from build123d import *

# Parameters (mm, degrees)
F1_DEPTH = 5
F3_DEPTH = 3
F4_W     = 12
F4_H     = 8
F5_DEPTH = 3.5
F6_W     = 12
F6_H     = 8
F7_DEPTH = 2
F8_W     = 11.5
F8_H     = 1
F9_DEPTH = 2


with BuildPart() as f1:
    # F0 (on Top) → F1 (new body)
    with BuildSketch(Plane.XY):
        Polygon((-20, -5), (-20, -15), (20, -15), (20, -5), (50, -5), (50, 5), (20, 5), (20, 15), (-20, 15), (-20, 5), (-50, 5), (-50, -5), align=None)
    extrude(amount=F1_DEPTH)

    # F2 (on face) → F3 (cut)
    with BuildSketch(Plane.XY.offset(5)):
        Polygon((16.5, 11), (-16.5, 11), (-16.5, 4), (-14.5, 4), (-14.5, -4), (-16.5, -4), (-16.5, -11), (16.5, -11), (16.5, -4), (14.5, -4), (14.5, 4), (16.5, 4), align=None)
    extrude(amount=-F3_DEPTH, mode=Mode.SUBTRACT)

    # F4 (on face) → F5 (cut)
    with BuildSketch(Plane.XY.offset(5)):
        with Locations((-20.5, 0)):
            Rectangle(F4_W, F4_H)
        with Locations((20.5, 0)):
            Rectangle(F4_W, F4_H)
    extrude(amount=-F5_DEPTH, mode=Mode.SUBTRACT)

    # F6 (on face) → F7 (cut)
    with BuildSketch(Plane.XY.offset(5)):
        with Locations((-32.5, 0)):
            Rectangle(F6_W, F6_H)
        with Locations((32.5, 0)):
            Rectangle(F6_W, F6_H)
    extrude(amount=-F7_DEPTH, mode=Mode.SUBTRACT)

    # F8 (on face) → F9 (cut)
    with BuildSketch(Plane.XY.offset(5)):
        with Locations((-44.25, 0)):
            Rectangle(F8_W, F8_H)
        with Locations((44.25, 0)):
            Rectangle(F8_W, F8_H)
    extrude(amount=-F9_DEPTH, mode=Mode.SUBTRACT)


solid = f1.part
Part model, mm, in its own coordinate system. A direction names the side the tool comes from. Give positions to 0.01 mm unless a question says otherwise; leave off trailing zeros. Loops run counter-clockwise (first coordinate to the right, second up) from the corner with the lowest first, then second, coordinate; pieces in that order, holes last. Notation, with made-up numbers: (-6, 11) -> (16, 11) arc R19 cw to (16, 15) -> close; hole circle Ø11 at (-25.75, 50). An arc over 180 degrees is marked (long way). Write each question's results on one line, items separated by ' | '. Start each with the question number.
Q1. Wall check: L1, parallel to X at y = -1.5, z = 2.95; L2, parallel to Y at x = 26, z = 3.7; L3, parallel to X at y = 6.75, z = 2.4. Give the ranges that are in metal, low to high.
Q2. Pull direction Y, two halves, no side cores. Call faces 1 (the face through (-35, -5, 2)), 2 (the face through (-16.5, 8, 4)), 3 (the face through (-20, 10, 2)): +Y half, -Y half, draft (parallel to the pull), parting line (faces both ways), or undercut.
Q3. Which spindle directions (+Z, -Z, +X, -X, +Y, -Y) get a long thin tool onto all of the face, cutting with end or side? Do faces 4 (the face through (-35, 5, 2)), 5 (the face through (50, 0, 2)), 6 (the face through (35, 5, 2)), 7 (the face through (44, 0.5, 4)), 8 (the face through (0, 0, 2)). Say none if no direction does.
Q4. Band-saw the part on A-A on y = 7.25. List the corners of the cut face in (x, z).
Q5. Band-saw the part on C-C on y = 12.25. List the corners of the cut face in (x, z), plus the area to 3 significant figures.
Q6. Pin check, flat tips, straight feed: P1, Ø2.5, axis at y = -6, z = 4, coming from the +X side; P2, Ø2, axis at x = 37.5, z = 4, coming from the +Y side; P3, Ø2, axis at x = -3.5, y = 2.5, coming from the +Z side; P4, Ø2, axis at y = 9, z = 1, coming from the -X side. Stop position of each tip, or through.
Q7. Band-saw the part on B-B on x = 25. List the corners of the cut face in (y, z), plus the area to 3 significant figures.
Results are:
1) L1: x = -50 to -26.5, 26.5 to 50 | L2: y = -5 to -4, 4 to 5 | L3: x = -20 to -16.5, 16.5 to 20
2) face 1: -Y half | face 2: undercut | face 3: draft
3) face 4: +Z, -Z, -X, +Y | face 5: +Z, -Z, +X, +Y, -Y | face 6: +Z, -Z, +X, +Y | face 7: +Z, +X, -X | face 8: +Z
4) outline: (-20, 0) -> (20, 0) -> (20, 5) -> (16.5, 5) -> (16.5, 2) -> (-16.5, 2) -> (-16.5, 5) -> (-20, 5) -> close
5) outline: (-20, 0) -> (20, 0) -> (20, 5) -> (-20, 5) -> close | area: 200 mm²
6) P1: stops at x = 50 | P2: stops at y = 5 | P3: stops at z = 2 | P4: stops at x = -20
7) outline: (-5, 0) -> (5, 0) -> (5, 5) -> (4, 5) -> (4, 1.5) -> (-4, 1.5) -> (-4, 5) -> (-5, 5) -> close | area: 22.0 mm²
